from build123d import *

# Parameters (mm, degrees)
F1_DEPTH = 1.27
F3_W     = 1.27
F3_H     = 1.778
F4_DEPTH = 1.27


with BuildPart() as f1:
    # F0 (on Right) → F1 (new body, symmetric)
    with BuildSketch(Plane.YZ):
        Polygon((-13.97, 1.778), (-13.97, 0), (6.35, 0), (6.35, 7.62), (0, 7.62), (0, 5.842), align=None)
    extrude(amount=F1_DEPTH, both=True)

    # F3 (on offset) → F4 (cut)
    with BuildSketch(Plane.XY.offset(7.62)):
        with Locations((0, 3.175)):
            Rectangle(F3_W, F3_H)
    extrude(amount=-F4_DEPTH, mode=Mode.SUBTRACT)


solid = f1.part
The model under review builds one solid part; all positions refer to its coordinate system, in mm. A direction names the side the tool comes from. Give positions to 0.01 mm unless a question says otherwise; leave off trailing zeros. Order: outer loops, then holes, each group sorted by start corner. A loop starts at its lowest first (then second) coordinate and runs counter-clockwise, first axis right, second up. Notation, with made-up numbers: M 78,-5 L 106,-5 A22 ccw 106,28 Z; hole C 14.25,15.25 d2. An arc over 180 degrees is marked long. Use one line per item in the form item = value. Start each with the question number.
Item 1: To check wall thickness, follow line 1 along Y through (x, z) = (-0.1, 7.25); line 2 along Y through (x, z) = (-1, 6.5); line 3 along Z through (x, y) = (0.85, -11.75). State the ranges of each line that lie inside material, in increasing order. Write a range as from..to.
Item 2: We need section C-C on z = 4.25. Give the boundary of the cut face in (x, y), plus the area to 3 significant figures.
Item 3: Insertion check: pin 1 Ø0.6 at (x, y) = (0, 3.5) entering from +Z; pin 2 Ø1.4 at (x, z) = (-0.5, 7) entering from -Y. Each pin has a flat end and moves straight along its axis. Give the tip position at first contact, or say it passes through.
Item 4: For faces 5 (the flat face through (0, 0, 7)), 6 (the flat face through (0.635, 3, 7)), 7 (the flat face through (0, -4, 0)), list the 3-axis set-ups (+Z, -Z, +X, -X, +Y, -Y) from which the entire face can be reached by the end or side of a thin tool; tool diameter is ignored.
Item 5: The part is to be moulded in two halves that separate along Y. For faces 1 (the flat face through (0, -13.97, 1)), 2 (the flat face through (0, 2.286, 7)), 3 (the flat face through (-1.27, -2, 3)), 4 (the flat face through (-0.635, 3, 7)), say which applies: pulls with the +Y half, pulls with the -Y half, needs draft (parallel to the pull), parting line crosses it, or undercut.
Item 6: We need section D-D on y = -6.75. Give the boundary of the cut face in (x, z).
Item 7: We need section B-B on x = 0.3. Give the boundary of the cut face in (y, z), plus the area to 3 significant figures.
Item 8: We need section A-A on y = 3.5. Give the boundary of the cut face in (x, z) (3 decimals).
Completed:
q1.line_1 = 0..2.29, 4.06..6.35
q1.line_2 = 0..6.35
q1.line_3 = 0..2.42
q2.outline = M -1.27,-5.47 L 1.27,-5.47 L 1.27,6.35 L -1.27,6.35 Z
q2.area = 30.0 mm²
q3.pin_1 = 6.35
q3.pin_2 = 0
q4.face_5 = +Z, +X, -X, -Y
q4.face_6 = +Z
q4.face_7 = -Z, +X, -X, +Y, -Y
q5.face_1 = pulls with the -Y half
q5.face_2 = undercut
q5.face_3 = needs draft
q5.face_4 = undercut
q6.outline = M -1.27,0 L 1.27,0 L 1.27,3.88 L -1.27,3.88 Z
q7.outline = M -13.97,0 L 6.35,0 L 6.35,7.62 L 4.06,7.62 L 4.06,6.35 L 2.29,6.35 L 2.29,7.62 L 0,7.62 L 0,5.84 L -13.97,1.78 Z
q7.area = 99.4 mm²
q8.outline = M -1.27,0 L 1.27,0 L 1.27,7.62 L 0.635,7.62 L 0.635,6.35 L -0.635,6.35 L -0.635,7.62 L -1.27,7.62 Z
